Here's how the part is built. I have some questions about the finished solid (model axes, mm). A direction names the side the tool comes from. Give positions to 0.01 mm unless a question says otherwise; leave off trailing zeros. Loops run counter-clockwise (first coordinate to the right, second up) from the corner with the lowest first, then second, coordinate; pieces in that order, holes last. Notation, with made-up numbers: M 27.5,15 L 56.5,15 A20 ccw 56.5,52 Z; hole C -11.5,33 d2. An arc over 180 degrees is marked long. Answer as CSV lines item,"result". Start each with the question number.
Item 1: I want a section at D-D on x = 51.5. List the corners of the cut face in (y, z) for me, plus the area to 3 significant figures.
Item 2: For faces 1 (the flat face through (131, -18, 90)), 2 (the flat face through (201, -17, 47)), which set-ups out of +Z, -Z, +X, -X, +Y, -Y let a thin tool reach every point of the face, with its end or its side?
Item 3: If we mould it in two halves opening along Z, with no side actions, what happens to faces 3 (the cylindrical face through (189.6, -19.46, 24.76)), 4 (the flat face through (129, -14, 44)), 5 (the flat face through (131, -18, 0))? For each: released by +Z, released by -Z, zero draft, split by the parting line, or undercut.
Item 4: I want a section at A-A on x = 176.7. List the corners of the cut face in (y, z) for me.
Item 5: Will these pins go through, and if not, where does the flat tip stop? P1, Ø3, axis at x = 207, z = 2.5, coming from the -Y side; P2, Ø5.5, axis at x = 51.5, z = 2.5, coming from the -Y side; P3, Ø0.8, axis at x = 112, y = -22.5, coming from the +Z side.
Item 6: I want a section at B-B on z = 87.5. List the corners of the cut face in (x, y) for me, plus the area to 3 significant figures.
Item 7: If I drill on line 1 along X through (y, z) = (-16.5, 2.5); line 2 along Z through (x, y) = (82.5, -16.25); line 3 along Z through (x, y) = (215, -18), over which ranges is the centre line in solid material (lowest first)? Write a range as from..to.
Item 8: I want a section at C-C on z = 45. List the corners of the cut face in (x, y) for me, plus the area to 3 significant figures.
from build123d import *

# Parameters (mm, degrees)
BOSS_EXTRUDE1_DEPTH   = 90
SKETCH2_R             = 24
CUT_EXTRUDE1_DEPTH    = 9
SKETCH3_R             = 25.1
CUT_EXTRUDE2_DEPTH    = 3
SKETCH4_W             = 143.5
SKETCH4_H             = 1
BOSS_EXTRUDE2_DEPTH   = 1
SKETCH5_W             = 10
SKETCH5_H             = 1
BOSS_EXTRUDE3_DEPTH   = 2
SKETCH6_R             = 1.65
CUT_EXTRUDE3_DEPTH    = 39
M3_TAPPED_HOLE1_D     = 2.5
M3_TAPPED_HOLE1_DEPTH = 8.5
M3_TAPPED_HOLE1_TIP   = 0.751075774
SKETCH_1_W            = 53.5
SKETCH_1_H            = 19
CUT_EXTRUDE_1_DEPTH   = 90


with BuildPart() as part:
    # Sketch1 → Boss-Extrude1 (new body)
    with BuildSketch(Plane.XY):
        Polygon((0, 0), (0, 5), (53.5, 5), (53.5, -14), (217, -14), (217, -22), (43.5, -22), (43.5, 0), align=None)
    extrude(amount=BOSS_EXTRUDE1_DEPTH)

    # Sketch2 → Cut-Extrude1 (cut, through all)
    with BuildSketch(Plane(origin=(0, -14, 0), x_dir=(1, 0, 0), z_dir=(0, 1, 0))):
        with Locations((176.7, -45)):
            Circle(SKETCH2_R)
    extrude(amount=-CUT_EXTRUDE1_DEPTH, mode=Mode.SUBTRACT)

    # Sketch3 → Cut-Extrude2 (cut)
    with BuildSketch(Plane(origin=(0, -14, 0), x_dir=(1, 0, 0), z_dir=(0, 1, 0))):
        with Locations((176.7, -45)):
            Circle(SKETCH3_R)
    extrude(amount=-CUT_EXTRUDE2_DEPTH, mode=Mode.SUBTRACT)

    # Sketch4 → Boss-Extrude2 (add)
    with BuildSketch(Plane.XZ.offset(22)):
        with Locations((145.25, 84.5)):
            Rectangle(SKETCH4_W, SKETCH4_H)
        with Locations((145.25, 5.5)):
            Rectangle(SKETCH4_W, SKETCH4_H)
    extrude(amount=BOSS_EXTRUDE2_DEPTH)

    # Sketch5 → Boss-Extrude3 (add)
    with BuildSketch(Plane.XZ):
        with Locations((28.5, 84.5)):
            Rectangle(SKETCH5_W, SKETCH5_H)
        with Locations((28.5, 5.5)):
            Rectangle(SKETCH5_W, SKETCH5_H)
    extrude(amount=BOSS_EXTRUDE3_DEPTH)

    # Sketch6 → Cut-Extrude3 (cut, through all)
    with BuildSketch(Plane(origin=(0, 15, 0), x_dir=(1, 0, 0), z_dir=(0, 1, 0))):
        with Locations((51.5, -2.5)):
            Circle(SKETCH6_R)
        with Locations((82.5, -2.5)):
            Circle(SKETCH6_R)
        with Locations((51.5, -87.5)):
            Circle(SKETCH6_R)
        with Locations((82.5, -87.5)):
            Circle(SKETCH6_R)
        with Locations((107, -87.5)):
            Circle(SKETCH6_R)
        with Locations((157, -87.5)):
            Circle(SKETCH6_R)
        with Locations((207, -87.5)):
            Circle(SKETCH6_R)
        with Locations((107, -2.5)):
            Circle(SKETCH6_R)
        with Locations((157, -2.5)):
            Circle(SKETCH6_R)
        with Locations((207, -2.5)):
            Circle(SKETCH6_R)
    extrude(amount=-CUT_EXTRUDE3_DEPTH, mode=Mode.SUBTRACT)

    # M3 Tapped Hole1
    with Locations(Plane(origin=(217, 0, 0), x_dir=(0, 0, -1), z_dir=(1, 0, 0))):
        with Locations((-70, -18), (-20, -18)):
            Hole(M3_TAPPED_HOLE1_D / 2, depth=M3_TAPPED_HOLE1_DEPTH)
            with Locations((0, 0, -(M3_TAPPED_HOLE1_DEPTH + M3_TAPPED_HOLE1_TIP / 2))):  # 118° drill point
                Cone(0, M3_TAPPED_HOLE1_D / 2, M3_TAPPED_HOLE1_TIP, mode=Mode.SUBTRACT)

    # 草图1 → 切除-拉伸1 (cut)
    with BuildSketch(Plane.XY.offset(90)):
        with Locations((26.75, -4.5)):
            Rectangle(SKETCH_1_W, SKETCH_1_H)
    extrude(amount=-CUT_EXTRUDE_1_DEPTH, mode=Mode.SUBTRACT)


solid = part.part
Result:
1,outline,"M -22,0 L -14,0 L -14,0.85 L -22,0.85 Z; M -22,4.15 L -14,4.15 L -14,85.85 L -22,85.85 Z; M -22,89.15 L -14,89.15 L -14,90 L -22,90 Z"
1,area,"667 mm^2"
2,face 1,"+Z, +X, -X, +Y, -Y"
2,face 2,"+Y"
3,face 3,"undercut"
3,face 4,"zero draft"
3,face 5,"released by -Z"
4,outline,"M -23,5 L -22,5 L -22,0 L -14,0 L -14,19.9 L -17,19.9 L -17,21 L -22,21 L -22,6 L -23,6 Z; M -23,84 L -22,84 L -22,69 L -17,69 L -17,70.1 L -14,70.1 L -14,90 L -22,90 L -22,85 L -23,85 Z"
5,P1,"through"
5,P2,"y = -22"
5,P3,"z = 85"
6,outline,"M 43.5,-22 L 49.85,-22 L 49.85,-14 L 43.5,-14 Z; M 53.15,-22 L 80.85,-22 L 80.85,-14 L 53.15,-14 Z; M 84.15,-22 L 105.35,-22 L 105.35,-14 L 84.15,-14 Z; M 108.65,-22 L 155.35,-22 L 155.35,-14 L 108.65,-14 Z; M 158.65,-22 L 205.35,-22 L 205.35,-14 L 158.65,-14 Z; M 208.65,-22 L 217,-22 L 217,-14 L 208.65,-14 Z"
6,area,"1,260 mm^2"
7,line 1,"43.5..49.85, 53.15..80.85, 84.15..105.35, 108.65..155.35, 158.65..205.35, 208.65..217"
7,line 2,"0..0.85, 4.15..85.85, 89.15..90"
7,line 3,"0..18.75, 21.25..68.75, 71.25..90"
8,outline,"M 43.5,-22 L 152.7,-22 L 152.7,-17 L 151.6,-17 L 151.6,-14 L 43.5,-14 Z; M 200.7,-22 L 217,-22 L 217,-14 L 201.8,-14 L 201.8,-17 L 200.7,-17 Z"
8,area,"997 mm^2"
